For this review, use the dimensioned drawing (mm, ordinates from the lowest corner) and the shaded views. A direction names the side the tool comes from. Round coordinates to 2 decimals unless told otherwise and drop trailing zeros. Loops run counter-clockwise (first coordinate to the right, second up) from the corner with the lowest first, then second, coordinate; pieces in that order, holes last. Notation, with made-up numbers: M 44,43.5 L 49,43.5 A11 ccw 49,63.5 Z; hole C -19,28 d1. An arc over 180 degrees is marked long. Answer as a JSON object with one key per item and string values. Group by question number.
Item 1: To check wall thickness, follow line 1 (Y direction, x = 7, z = 11.5); line 2 (X direction, y = 5.5, z = 17.5); line 3 (Y direction, x = 68, z = 6) (3 decimals). State the ranges of each line that lie inside material, in increasing order.
Item 2: Insertion check: P1, Ø2, axis at x = 19, y = 15.5, coming from the +Z side; P2, Ø6.5, axis at y = 16, z = 9.5, coming from the -X side; P3, Ø1.5, axis at y = 18, z = 17.5, coming from the +X side; P4, Ø4, axis at x = 30.5, y = 4.5, coming from the -Z side. Each pin has a flat end and moves straight along its axis. Give the tip position at first contact, or say it passes through.
Item 3: Consider section D-D (x = 15). Give the boundary of the cut face in (y, z), and give its area (3 significant figures).
Item 4: Tool access review of the marked faces 1, 2 and 3: name each direction out of +Z, -Z, +X, -X, +Y, -Y from which nothing blocks a thin tool from reaching the whole face with its end or side.
Item 5: Consider section A-A (y = 11). Give the boundary of the cut face in (x, z).
Item 6: Consider section C-C (x = 35.5). Give the boundary of the cut face in (y, z), and give its area (3 significant figures).
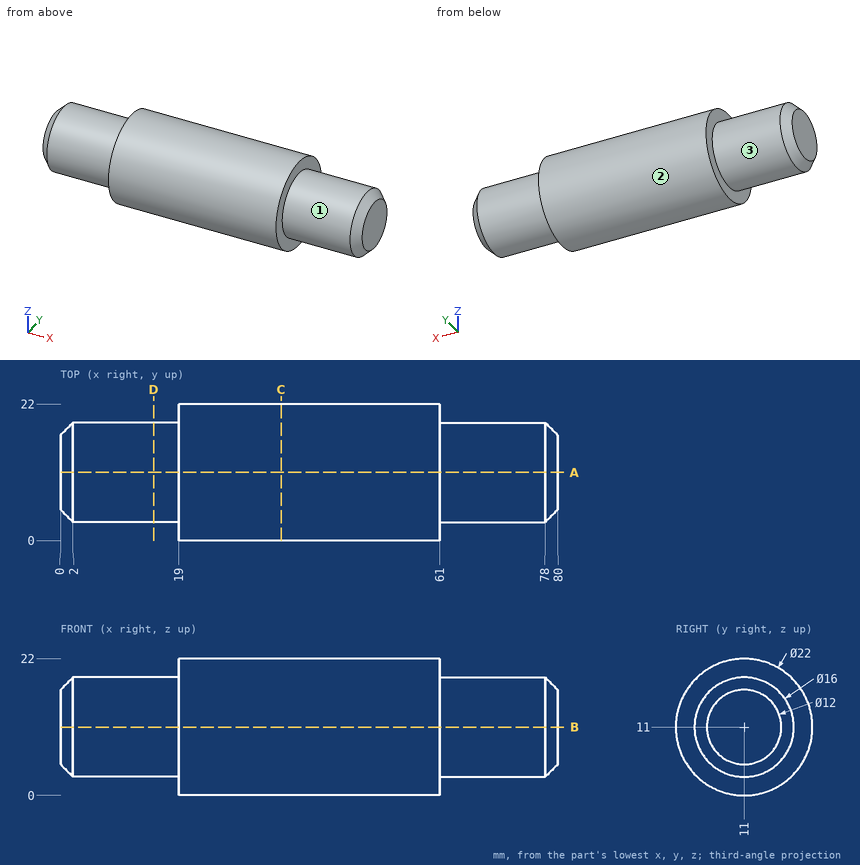
Geometry results:
{
 "1": {"line 1": "y = 3.02 to 18.98", "line 2": "x = 19 to 61", "line 3": "y = 4.755 to 17.245"},
 "2": {"P1": "stops at z = 21.43", "P2": "stops at x = 0", "P3": "stops at x = 61", "P4": "stops at z = 0.96"},
 "3": {"outline": "C 11,11 d16", "area": "201 mm^2"},
 "4": {"face 1": "+X", "face 2": "+X, -X", "face 3": "-X"},
 "5": {"outline": "M 0,5 L 2,3 L 19,3 L 19,0 L 61,0 L 61,3 L 78,3 L 80,5 L 80,17 L 78,19 L 61,19 L 61,22 L 19,22 L 19,19 L 2,19 L 0,17 Z"},
 "6": {"outline": "C 11,11 d22", "area": "380 mm^2"}
}
